Geometry check sheet. Reference: drawing and pictorial views, mm from the part's lowest x, y, z. Give positions to 0.01 mm unless a question says otherwise; leave off trailing zeros. Write each loop counter-clockwise with the first axis right and the second up, starting at its lowest first coordinate (ties: lowest second). Pieces come first, ordered by that corner, then holes. Notation, with made-up numbers: (27, -29) -> (73, -29) arc R12 ccw to (73, -14) -> close; hole circle Ø1 at (-38, 47.25). An arc over 180 degrees is marked (long way). Return JSON: item names as keys, results as strings.
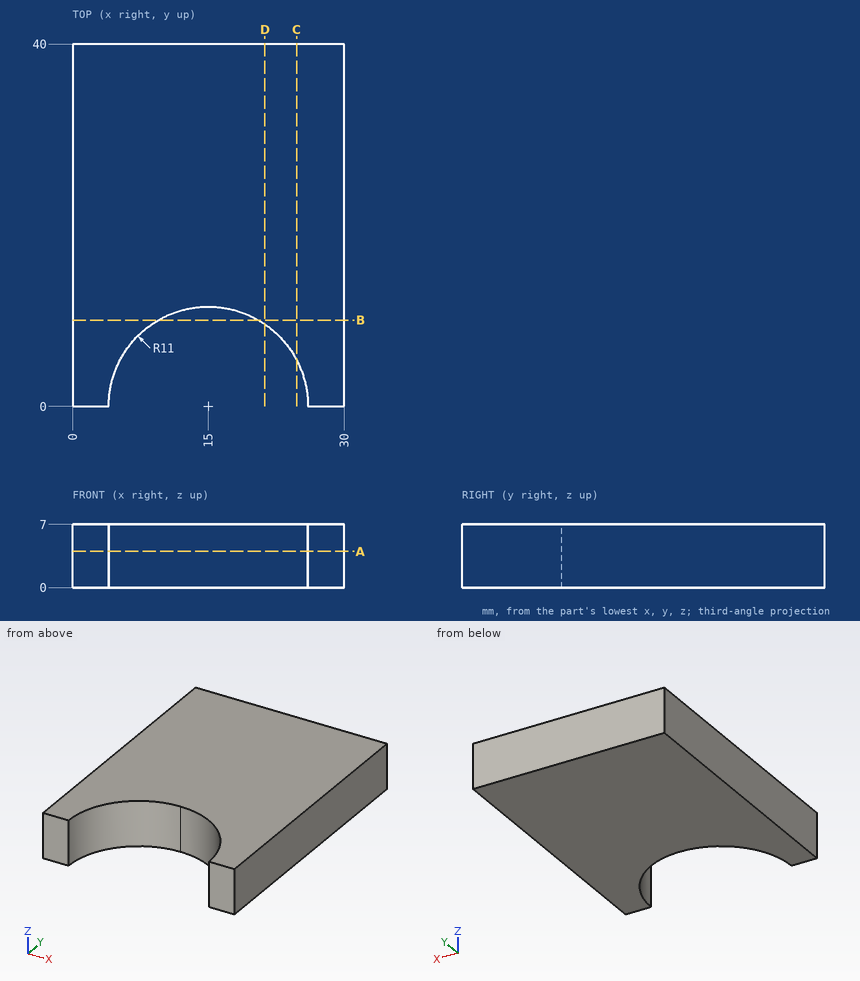
(1) Cross-section at A-A on z = 4. Enter the section's corners in (x, y), then the cut area to 3 significant figures.
Reply:
{"outline": "(0, 0) -> (4, 0) arc R11 cw to (15, 11) arc R11 cw to (26, 0) -> (30, 0) -> (30, 40) -> (0, 40) -> close", "area": "1,010 mm^2"}
(2) Cross-section at B-B on y = 9.5. Enter the section's corners in (x, z), then the cut area to 3 significant figures.
Reply:
{"outline": "(0, 0) -> (9.45, 0) -> (9.45, 7) -> (0, 7) -> close; (20.55, 0) -> (30, 0) -> (30, 7) -> (20.55, 7) -> close", "area": "132 mm^2"}
(3) Cross-section at D-D on x = 21.25. Enter the section's corners in (y, z), then the cut area to 3 significant figures.
Reply:
{"outline": "(9.05, 0) -> (40, 0) -> (40, 7) -> (9.05, 7) -> close", "area": "217 mm^2"}
(4) Thickness scan on L1, parallel to X at y = 7.5, z = 1.5; L2, parallel to X at y = 7, z = 3.5; L3, parallel to Y at x = 8, z = 0.75. Record the ranges inside material, lowest first.
Reply:
{"L1": "0 to 6.95, 23.05 to 30", "L2": "0 to 6.51, 23.49 to 30", "L3": "8.49 to 40"}
(5) Cross-section at C-C on x = 24.75. Enter the section's corners in (y, z), then the cut area to 3 significant figures.
Reply:
{"outline": "(5.09, 0) -> (40, 0) -> (40, 7) -> (5.09, 7) -> close", "area": "244 mm^2"}
